from build123d import *

# Parameters (mm, degrees)
SKETCH3_R           = 124.360538227
BOSS_EXTRUDE2_DEPTH = 80
SKETCH4_W           = 150
SKETCH4_H           = 80
BOSS_EXTRUDE4_DEPTH = 260
SKETCH5_R           = 20
CUT_EXTRUDE1_DEPTH  = 260
SKETCH6_W           = 50
SKETCH6_H           = 100
CUT_EXTRUDE2_DEPTH  = 260


with BuildPart() as part:
    # Sketch3 → Boss-Extrude2 (new body)
    with BuildSketch(Plane.XY):
        Circle(SKETCH3_R)
    extrude(amount=BOSS_EXTRUDE2_DEPTH)

    # Sketch4 → Boss-Extrude4 (add)
    with BuildSketch(Plane.XY):
        Rectangle(SKETCH4_W, SKETCH4_H)
    extrude(amount=BOSS_EXTRUDE4_DEPTH)

    # Sketch5 → Cut-Extrude1 (cut)
    with BuildSketch(Plane.ZY.offset(75)):
        with Locations((220, 0)):
            Circle(SKETCH5_R)
    extrude(amount=-CUT_EXTRUDE1_DEPTH, mode=Mode.SUBTRACT)

    # Sketch6 → Cut-Extrude2 (cut)
    with BuildSketch(Plane(origin=(0, 40, 0), x_dir=(1, 0, 0), z_dir=(0, 1, 0))):
        with Locations((0, -210)):
            Rectangle(SKETCH6_W, SKETCH6_H)
    extrude(amount=-CUT_EXTRUDE2_DEPTH, mode=Mode.SUBTRACT)


solid = part.part
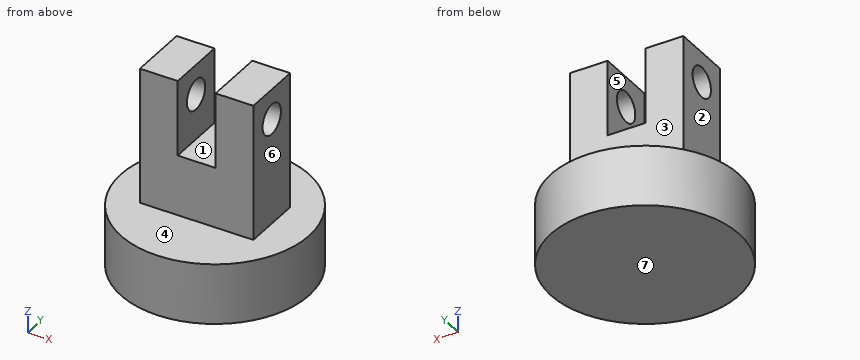
Model file for the job. Use its own axes, mm. Face numbers are marked on the shaded views. A direction names the side the tool comes from. Coordinates: 2 decimals unless noted, no trailing zeros. Order: outer loops, then holes, each group sorted by start corner. A loop starts at its lowest first (then second) coordinate and runs counter-clockwise, first axis right, second up. Notation, with made-up numbers: (-4, 83.25) -> (27, 83.25) arc R6 cw to (27, 89.25) -> close; hole circle Ø4 at (80.5, 77.5). An arc over 180 degrees is marked (long way). Return JSON: item names as keys, results as strings. Group by question number.
Item 1: Wall check: line 1 along Y through (x, z) = (-53, 220); line 2 along X through (y, z) = (38.5, 197); line 3 along Z through (x, y) = (-54, -1). Give the ranges that are in metal, low to high. Write a range as [from, to].
Item 2: Flat gauge pins, fed straight in: P1, Ø8, axis at y = -40.5, z = 107.5, coming from the -X side; P2, Ø5, axis at x = 11.5, z = 148.5, coming from the +Y side; P3, Ø12, axis at x = -53, y = -60.5, coming from the +Z side. Where does each tip first touch, or does it go through?
Item 3: Pull direction X, two halves, no side cores. Call the marked faces 5, 6 and 7: pulls with the +X half, pulls with the -X half, needs draft (parallel to the pull), parting line crosses it, or undercut.
Item 4: Saw through at B-B on y = 0. Write the cut outline in (x, z).
Item 5: Saw through at A-A on z = 220. Write the cut outline in (x, y).
Item 6: Tool access for the marked faces 1, 2, 3 and 4: list every direction of +Z, -Z, +X, -X, +Y, -Y with a clear straight run to the whole face (end or side of a thin tool).
Item 7: Saw through at D-D on x = -60.5. Write the cut outline in (y, z), then the cut area to 3 significant figures.
Item 8: Saw through at C-C on x = 0. Write the cut outline in (y, z), then the cut area to 3 significant figures.
Values found:
{
 "1": {"line 1": "y = [-40, -20], [20, 40]", "line 2": "x = [-75, -25], [25, 75]", "line 3": "z = [0, 200.03], [239.97, 260]"},
 "2": {"P1": "stops at x = -75", "P2": "stops at y = 40", "P3": "stops at z = 80"},
 "3": {"face 5": "undercut", "face 6": "pulls with the +X half", "face 7": "needs draft"},
 "4": {"outline": "(-124.36, 0) -> (124.36, 0) -> (124.36, 80) -> (75, 80) -> (75, 200) -> (25, 200) -> (25, 160) -> (-25, 160) -> (-25, 200) -> (-75, 200) -> (-75, 80) -> (-124.36, 80) -> close; (-75, 240) -> (-25, 240) -> (-25, 260) -> (-75, 260) -> close; (25, 240) -> (75, 240) -> (75, 260) -> (25, 260) -> close"},
 "5": {"outline": "(-75, -40) -> (-25, -40) -> (-25, -20) -> (-75, -20) -> close; (-75, 20) -> (-25, 20) -> (-25, 40) -> (-75, 40) -> close; (25, -40) -> (75, -40) -> (75, -20) -> (25, -20) -> close; (25, 20) -> (75, 20) -> (75, 40) -> (25, 40) -> close"},
 "6": {"face 1": "+Z, +Y, -Y", "face 2": "+Z, -X, +Y, -Y", "face 3": "+Z, +X, -X, +Y", "face 4": "+Z"},
 "7": {"outline": "(-108.65, 0) -> (108.65, 0) -> (108.65, 80) -> (40, 80) -> (40, 260) -> (-40, 260) -> (-40, 80) -> (-108.65, 80) -> close; hole circle Ø40 at (0, 220)", "area": "30,500 mm2"},
 "8": {"outline": "(-124.36, 0) -> (124.36, 0) -> (124.36, 80) -> (40, 80) -> (40, 160) -> (-40, 160) -> (-40, 80) -> (-124.36, 80) -> close", "area": "26,300 mm2"}
}
